For this review, take the finished solid that the model builds, in its own axes (mm). A direction names the side the tool comes from. Give positions to 0.01 mm unless a question says otherwise; leave off trailing zeros. Order: outer loops, then holes, each group sorted by start corner. A loop starts at its lowest first (then second) coordinate and runs counter-clockwise, first axis right, second up. Notation, with made-up numbers: M -26,-24.5 L 1,-24.5 A15 ccw 1,-2.5 Z; hole C 72.5,83.25 d1. An arc over 180 degrees is marked long. Use CSV: the item, a comma, the result in double quotes. Start each with the question number.
(1) Wall thickness on L1, parallel to Y at x = 0, z = -108; L2, parallel to Y at x = 0, z = -199.35; L3, parallel to X at y = 8.5, z = -122: over which ranges is each line inside the solid? List them lowest first. Write a range as from..to.
(2) Tool access review of faces 1 (the face through (-34, 0, 2)), 2 (the face through (-4.686, 35.694, -98.6)), 3 (the face through (-7.262, -32.703, -94.077)): name each direction out of +Z, -Z, +X, -X, +Y, -Y from which nothing blocks a thin tool from reaching the whole face with its end or side.
(3) Draft analysis for pull direction X (two halves, no side actions). For faces 4 (the face through (-0.2, -36.3, 0)), 5 (the face through (-9, -40, 1)), 6 (the face through (22.878, 7.205, -197.014)), state which applies: pulls with the +X half, pulls with the -X half, needs draft (parallel to the pull), parting line crosses it, or undercut.
(4) Clearance check with flat-ended pins moving along their axes: P1, Ø10, axis at x = 16.5, z = -47, coming from the +Y side; P2, Ø10, axis at x = -9.5, z = -106, coming from the -Y side; P3, Ø5, axis at x = 4, z = -154.5, coming from the +Y side. State where each tip first meets the part, or that it passes through.
(5) Consider section C-C (z = -67.5). Write out the cut boundary in (x, y), and give its area (3 significant figures).
```python
from build123d import *

# Parameters (mm, degrees)
F0_R     = 41
F0_R_2   = 36
F1_DEPTH = 2
F2_DEPTH = 200
F3_T     = 2.5
F5_R     = 23.5
F6_DEPTH = 25
F7_SIZE  = 9.99999


# Not quite as in the source:
# - a fillet or chamfer is up to 0.001 mm smaller than in the source, because OpenCascade refuses the exact size
# - a shell that OpenCascade refuses in one call is made with other operations: the cavity is built on its own and cut out


with BuildPart() as f1:
    # F0 (on Top) → F1 (new body)
    with BuildSketch(Plane.XY):
        Circle(F0_R)
        Circle(F0_R_2, mode=Mode.SUBTRACT)
        Circle(F0_R_2)
    extrude(amount=F1_DEPTH)

    # F0 (on Top) → F2 (join)
    with BuildSketch(Plane.XY):
        Circle(F0_R_2)
    extrude(amount=-F2_DEPTH)

    # F3: shell of thickness 2.5, made by hand


with BuildPart() as f3_core1:
    # F3_t2: copy of F1
    add(f1.part)

    # the walls: a layer under each face that stays
    f3_faces = [f3_core1.faces().sort_by_distance(p)[0] for p in [
        (-41, 0, 1),
        (-27.3333333333, -27.3333333333, 0),
        (-36, 0, -100),
        (0, 0, -200),
    ]]
    thicken(f3_faces, amount=-F3_T, mode=Mode.SUBTRACT)

    # F3_s3 → F3_t4 (revolve, cut)
    with BuildSketch(Plane.XZ):
        Polygon((36.025, -0.025), (36, 2.5), (33.5, 2.5), (33.5, 0), align=None)
    revolve(axis=Axis((0, 0, 0), (0, 0, 1)), mode=Mode.SUBTRACT)


with BuildPart() as f1_1:
    add(f1.part)

    # what is left inside the walls is the cavity
    f3_cavity = [f3_core1.part.solids().sort_by_distance(p)[0] for p in [
        (-33.475, 0, -64.5),
    ]]
    add(f3_cavity, mode=Mode.SUBTRACT)

    # F5 (on offset) → F6 (cut)
    with BuildSketch(Plane(origin=(0, 0, -200), x_dir=(1, 0, 0), z_dir=(0, 0, -1))):
        Circle(F5_R)
    extrude(amount=-F6_DEPTH, mode=Mode.SUBTRACT)

    # F7 (size 10 in the source; OpenCascade refuses exactly that, so slightly less here)
    f7_edges = [f1_1.edges().sort_by_distance(p)[0] for p in [
        (33.5, 0, -97.75),
        (-33.5, 0, -197.5),
    ]]
    chamfer(f7_edges, length=F7_SIZE)


solid = f1_1.part
```
Check result:
1,L1,"y = -36..-33.5, 33.5..36"
1,L2,"y = -36..-23.5, 23.5..36"
1,L3,"x = -34.98..-32.4, 32.4..34.98"
2,face 1,"+Z, +X, -X, +Y, -Y"
2,face 2,"-Z"
2,face 3,"+Z"
3,face 4,"needs draft"
3,face 5,"parting line crosses it"
3,face 6,"undercut"
4,P1,"stops at y = 34.11"
4,P2,"stops at y = -35.72"
4,P3,"stops at y = 35.97"
5,outline,"C 0,0 d72; hole C 0,0 d67"
5,area,"546 mm^2"
